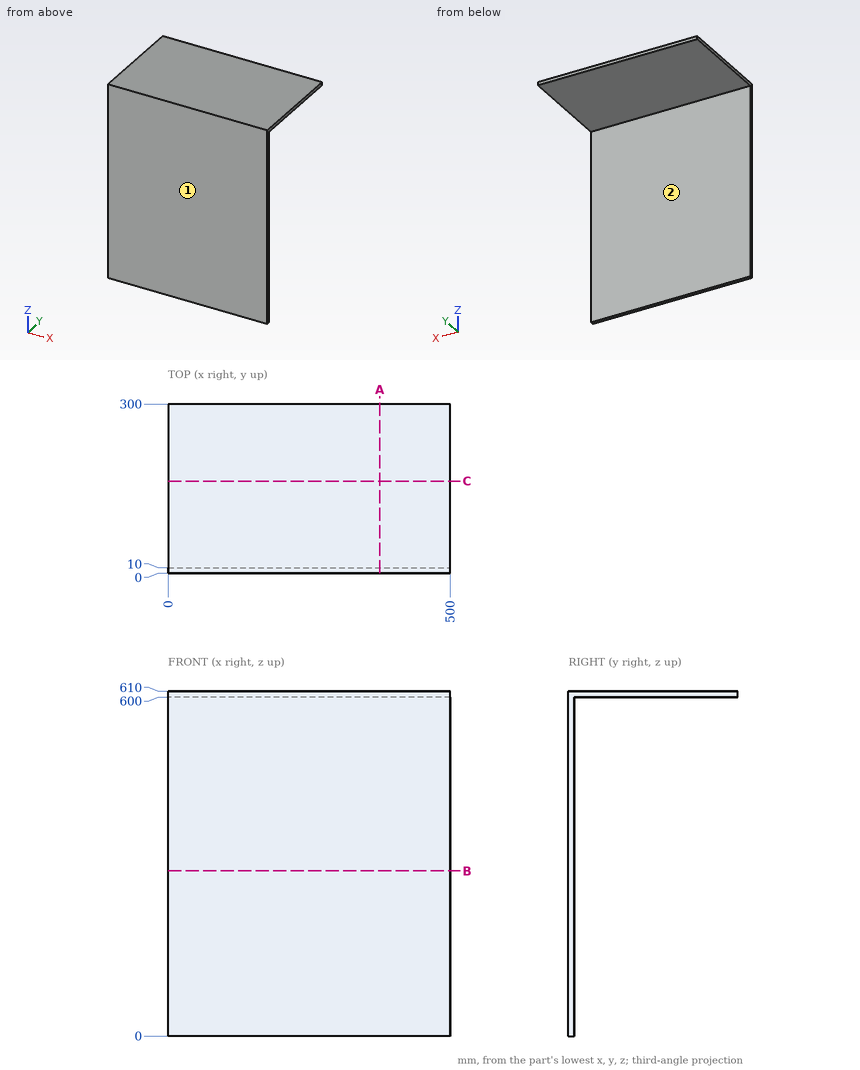
Could you check a few things on this drawing? It's one solid part, dimensions in mm from its lowest x, y, z. A direction names the side the tool comes from. Round coordinates to 2 decimals unless told otherwise and drop trailing zeros. Loops run counter-clockwise (first coordinate to the right, second up) from the corner with the lowest first, then second, coordinate; pieces in that order, holes last.
Q1. Please list where these lines run through material, in increasing order: L1, parallel to Y at x = 176, z = 34; L2, parallel to Z at x = 477, y = 74.5.
Q2. I want a section at A-A (x = 375). Write out the boundary of the cut face in (y, z), and give its area (3 significant figures).
Q3. I want a section at B-B (z = 292.5). Write out the boundary of the cut face in (x, y).
Q4. For P1, Ø10, axis at x = 341, y = 213, coming from the -Z side; P2, Ø6, axis at x = 173, z = 116, coming from the +Y side, each with a flat end and sliding along its axis, tell me the tip position at first contact or that it passes through.
Q5. On a 3-axis mill with a long thin cutter (end or side, diameter ignored), from which of +Z, -Z, +X, -X, +Y, -Y can I reach the whole of each face in a straight line? I mean the marked faces 1 and 2. Say none if no direction works.
Q6. I want a section at C-C (y = 163.5). Write out the boundary of the cut face in (x, z).
Answer below:
1. L1: y = 0 to 10
1. L2: z = 600 to 610
2. outline: (0, 0) - (10, 0) - (10, 600) - (300, 600) - (300, 610) - (0, 610) - close
2. area: 9,000 mm2
3. outline: (0, 0) - (500, 0) - (500, 10) - (0, 10) - close
4. P1: stops at z = 600
4. P2: stops at y = 10
5. face 1: +Z, -Z, +X, -X, -Y
5. face 2: -Z, +X, -X, +Y
6. outline: (0, 600) - (500, 600) - (500, 610) - (0, 610) - close
